Geometry: see drawing. Coordinates: mm, zero at the bounding-box minimum. Coordinates: 2 decimals unless noted, no trailing zeros. Order: outer loops, then holes, each group sorted by start corner. A loop starts at its lowest first (then second) coordinate and runs counter-clockwise, first axis right, second up.
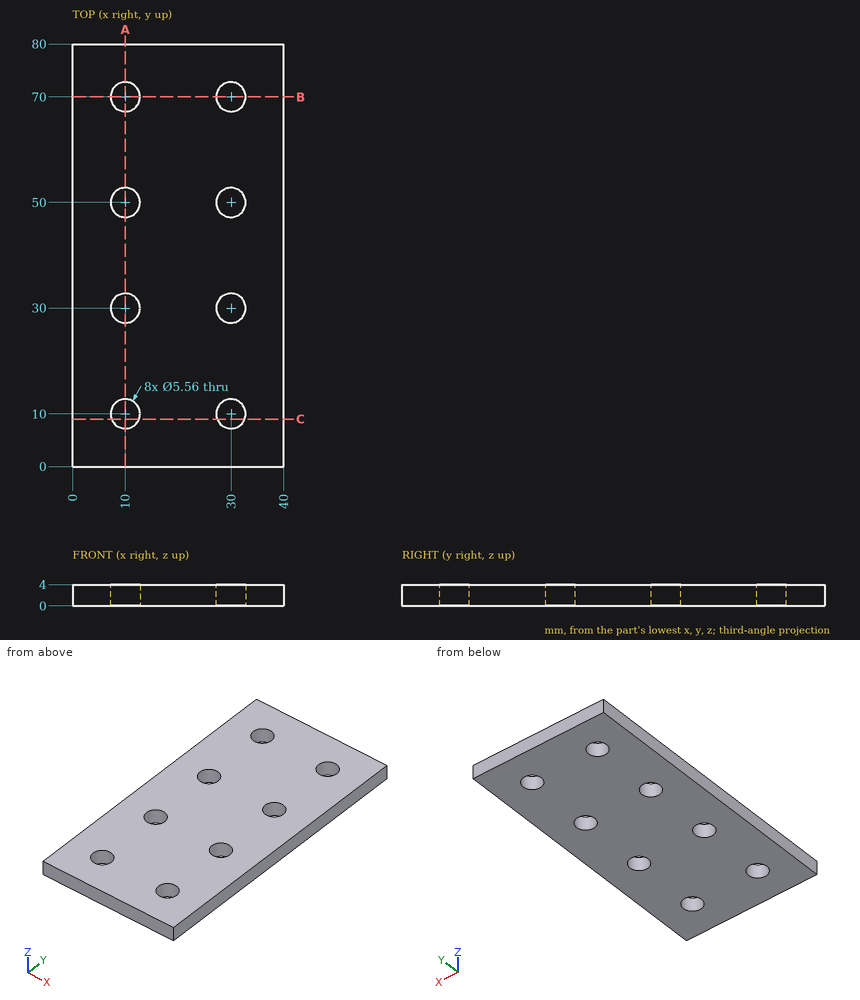
Item 1: Cut plane B-B on y = 70. Return loops of the section in (x, z).
Response values:
outline: (0, 0) - (7.22, 0) - (7.22, 4) - (0, 4) - close; (12.78, 0) - (27.22, 0) - (27.22, 4) - (12.78, 4) - close; (32.78, 0) - (40, 0) - (40, 4) - (32.78, 4) - close
Item 2: Cut plane C-C on y = 9. Return loops of the section in (x, z), then the cut area to 3 significant figures.
Response values:
outline: (0, 0) - (7.41, 0) - (7.41, 4) - (0, 4) - close; (12.59, 0) - (27.41, 0) - (27.41, 4) - (12.59, 4) - close; (32.59, 0) - (40, 0) - (40, 4) - (32.59, 4) - close
area: 118 mm2
Item 3: Cut plane A-A on x = 10. Return loops of the section in (y, z), then the cut area to 3 significant figures.
Response values:
outline: (0, 0) - (7.22, 0) - (7.22, 4) - (0, 4) - close; (12.78, 0) - (27.22, 0) - (27.22, 4) - (12.78, 4) - close; (32.78, 0) - (47.22, 0) - (47.22, 4) - (32.78, 4) - close; (52.78, 0) - (67.22, 0) - (67.22, 4) - (52.78, 4) - close; (72.78, 0) - (80, 0) - (80, 4) - (72.78, 4) - close
area: 231 mm2
Item 4: Ray query, probe 1 along Y at (x, z) = (30, 2.2); probe 2 along X at (y, z) = (11.5, 2.6); probe 3 along Y at (x, z) = (30.5, 3.3). Return the intervals inside material, ascending.
Response values:
probe 1: y = 0 to 7.22, 12.78 to 27.22, 32.78 to 47.22, 52.78 to 67.22, 72.78 to 80
probe 2: x = 0 to 7.66, 12.34 to 27.66, 32.34 to 40
probe 3: y = 0 to 7.27, 12.73 to 27.27, 32.73 to 47.27, 52.73 to 67.27, 72.73 to 80
